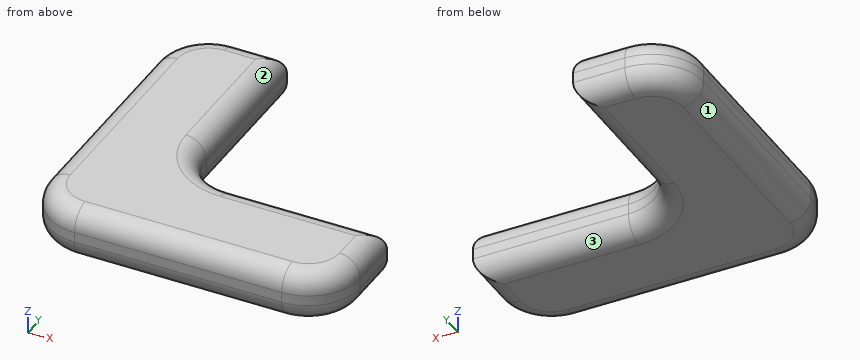
from build123d import *

# Parameters (mm, degrees)
SKETCH1_W           = 10
SKETCH1_H           = 10
BOSS_EXTRUDE1_DEPTH = 5
SKETCH2_W           = 10
SKETCH2_H           = 5
BOSS_EXTRUDE2_DEPTH = 20
SKETCH3_W           = 5
SKETCH3_H           = 10
BOSS_EXTRUDE3_DEPTH = 20
FILLET1_R           = 5
FILLET2_R           = 2


with BuildPart() as part:
    # Sketch1 → Boss-Extrude1 (new body)
    with BuildSketch(Plane.XY):
        with Locations((5, -5)):
            Rectangle(SKETCH1_W, SKETCH1_H)
    extrude(amount=BOSS_EXTRUDE1_DEPTH)

    # Sketch2 → Boss-Extrude2 (add)
    with BuildSketch(Plane(origin=(0, 0, 0), x_dir=(1, 0, 0), z_dir=(0, 1, 0))):
        with Locations((5, -2.5)):
            Rectangle(SKETCH2_W, SKETCH2_H)
    extrude(amount=BOSS_EXTRUDE2_DEPTH)

    # Sketch3 → Boss-Extrude3 (add)
    with BuildSketch(Plane(origin=(10, 0, 0), x_dir=(0, 0, -1), z_dir=(1, 0, 0))):
        with Locations((-2.5, -5)):
            Rectangle(SKETCH3_W, SKETCH3_H)
    extrude(amount=BOSS_EXTRUDE3_DEPTH)

    # Fillet1
    fillet1_edges = [part.edges().sort_by_distance(p)[0] for p in [
        (0, 20, 2.5),
        (10, 0, 2.5),
        (30, -10, 2.5),
        (0, -10, 2.5),
    ]]
    fillet(fillet1_edges, radius=FILLET1_R)

    # Fillet2
    fillet2_edges = [part.edges().sort_by_distance(p)[0] for p in [
        (7.5, 20, 0),
        (22.5, 0, 5),
        (22.5, 0, 0),
        (30, -2.5, 5),
        (30, -2.5, 0),
        (0, 5, 0),
        (10, 12.5, 0),
        (15, -10, 0),
        (1.464466094, -8.535533906, 0),
        (1.464466094, 18.535533906, 0),
        (28.535533906, -8.535533906, 0),
        (15, -10, 5),
        (0, 5, 5),
        (10, 12.5, 5),
        (7.5, 20, 5),
        (1.464466094, -8.535533906, 5),
        (1.464466094, 18.535533906, 5),
        (28.535533906, -8.535533906, 5),
        (11.464466094, 1.464466094, 5),
        (11.464466094, 1.464466094, 0),
    ]]
    fillet(fillet2_edges, radius=FILLET2_R)


solid = part.part
The model under review builds one solid part; all positions refer to its coordinate system, in mm. Face numbers are marked on the shaded views. A direction names the side the tool comes from. Round coordinates to 2 decimals unless told otherwise and drop trailing zeros. Order: outer loops, then holes, each group sorted by start corner. A loop starts at its lowest first (then second) coordinate and runs counter-clockwise, first axis right, second up. Notation, with made-up numbers: (89.25, 46) -> (105.25, 46) arc R16 cw to (105.25, 65) -> close; hole circle Ø4 at (83.5, -4.5). An arc over 180 degrees is marked (long way). Return JSON: item names as keys, results as strings.
1. Take a section at C-C (x = 19.5). Write out the cut boundary in (y, z).
Answer block:
{"outline": "(-10, 2) arc R2 ccw to (-8, 0) -> (-2, 0) arc R2 ccw to (0, 2) -> (0, 3) arc R2 ccw to (-2, 5) -> (-8, 5) arc R2 ccw to (-10, 3) -> close"}
2. For L1, parallel to X at y = 11, z = 2.9; L2, parallel to X at y = 17.5, z = 1.5; L3, parallel to Y at x = 19.25, z = 0.4, list the stretches that pass through material, from the lowest coordinate up. Write a range as [from, to].
Answer block:
{"L1": "x = [0, 10]", "L2": "x = [0.74, 9.94]", "L3": "y = [-9.2, -0.8]"}
3. Take a section at B-B (y = -4). Write out the cut boundary in (x, z), then the cut area to 3 significant figures.
Answer block:
{"outline": "(0, 2) arc R2 ccw to (2, 0) -> (28, 0) arc R2 ccw to (30, 2) -> (30, 3) arc R2 ccw to (28, 5) -> (2, 5) arc R2 ccw to (0, 3) -> close", "area": "147 mm²"}
4. Insertion check: P1, Ø2, axis at x = 12, z = 1, coming from the +Y side; P2, Ø1.1, axis at y = 10.5, z = 2.5, coming from the +X side; P3, Ø2, axis at x = 26.5, z = 4, coming from the +Y side. Each pin has a flat end and moves straight along its axis. Give the tip position at first contact, or say it passes through.
Answer block:
{"P1": "stops at y = 1.75", "P2": "stops at x = 10", "P3": "stops at y = 0"}
5. Take a section at D-D (z = 2.5). Write out the cut boundary in (x, y).
Answer block:
{"outline": "(0, -5) arc R5 ccw to (5, -10) -> (25, -10) arc R5 ccw to (30, -5) -> (30, 0) -> (15, 0) arc R5 cw to (10, 5) -> (10, 20) -> (5, 20) arc R5 ccw to (0, 15) -> close"}
6. For the marked faces 1, 2 and 3, list the 3-axis set-ups (+Z, -Z, +X, -X, +Y, -Y) from which the entire face can be reached by the end or side of a thin tool; tool diameter is ignored.
Answer block:
{"face 1": "-Z, -X, +Y, -Y", "face 2": "+Z, +X, +Y", "face 3": "-Z, +X, +Y"}
7. Take a section at A-A (z = 4.2). Write out the cut boundary in (x, y), then the cut area to 3 significant figures.
Answer block:
{"outline": "(0.4, -5) arc R4.6 ccw to (5, -9.6) -> (25, -9.6) arc R4.6 ccw to (29.6, -5) -> (29.6, -0.4) -> (15, -0.4) arc R5.4 cw to (9.6, 5) -> (9.6, 19.6) -> (5, 19.6) arc R4.6 ccw to (0.4, 15) -> close", "area": "445 mm²"}
